Can you work these out from the model? Positions are in its coordinate system, mm. Face numbers are marked on the shaded views. A direction names the side the tool comes from. Give positions to 0.01 mm unless a question says otherwise; leave off trailing zeros. Loops run counter-clockwise (first coordinate to the right, second up) from the corner with the lowest first, then second, coordinate; pieces in that order, holes last. Notation, with made-up numbers: M 54.5,74.5 L 71.5,74.5 A35 ccw 71.5,110.5 Z; hole C 70.25,19 d8. An arc over 180 degrees is marked long. Put each result on its own line as item: value. Start each with the question number.
1) For the marked faces 5, 6 and 7, which set-ups out of +Z, -Z, +X, -X, +Y, -Y let a thin tool reach every point of the face, with its end or its side?
2) Please list where these lines run through material, in increasing order: line 1 along Y through (x, z) = (15, 7); line 2 along X through (y, z) = (58.75, 2.75); line 3 along X through (y, z) = (58.25, 8.5). Write a range as from..to.
3) Imagine slicing it at C-C (z = 15). State how many separate pieces and enclosed holes the cut face has, then the cut area to 3 significant figures.
4) Imagine slicing it at B-B (x = 15). Write out the boundary of the cut face in (y, z), then the cut area to 3 significant figures.
5) Imagine slicing it at A-A (x = -15). Write out the boundary of the cut face in (y, z), then the cut area to 3 significant figures.
6) Imagine slicing it at D-D (x = -9). Write out the boundary of the cut face in (y, z).
7) If we mould it in two halves opening along Y, with no side actions, what happens to the marked faces 1, 2, 3 and 4? For each: +Y half, -Y half, draft (parallel to the pull), parting line (faces both ways), or undercut.
8) For P1, Ø5, axis at x = 17.5, z = 11, coming from the +Y side; P2, Ø8, axis at x = 13, y = 59.5, coming from the -Z side; P3, Ø8, axis at x = 26, y = 58, coming from the +Z side; P4, Ø4, axis at x = 12.5, z = 6, coming from the -Y side, each with a flat end and sliding along its axis, tell me the tip position at first contact or that it passes through.
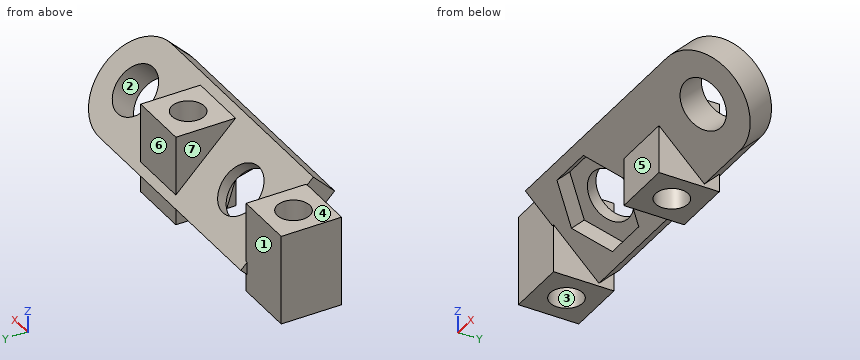
from build123d import *

# Parameters (mm, degrees)
SKETCH039_R             = 4.2
PAD019_DEPTH            = 5
BOX_W                   = 10
BOX_H                   = 10
BOX_DEPTH               = 15
POCKET011_DEPTH         = 3
SKETCH041_R             = 2.7
POCKET012_DEPTH         = 130.641501891
BODY007_PLACEMENT_ANGLE = 45


with BuildPart() as part:
    # Sketch039 → Pad019 (new body)
    with BuildSketch(Plane.XZ):
        with BuildLine():
            ThreePointArc((30, -8.5), (38.5, 0), (30, 8.5))
            Line((0, 8.5), (30, 8.5))
            Line((-10.313604, 8.5), (0, 8.5))
            Line((-10.313604, -8.5), (-10.313604, 8.5))
            Line((0, -8.5), (-10.313604, -8.5))
            Line((0, -8.5), (30, -8.5))
        make_face()
        Circle(SKETCH039_R, mode=Mode.SUBTRACT)
        with Locations((30, 0)):
            Circle(SKETCH039_R, mode=Mode.SUBTRACT)
    extrude(amount=PAD019_DEPTH)

    # Box → Box (join)
    with BuildSketch(Plane(origin=(10, 7, 0), x_dir=(1, 0, 0), z_dir=(0, -0.7071067812, -0.7071067812))):
        with Locations((5, 5)):
            Rectangle(BOX_W, BOX_H)
    box = extrude(amount=BOX_DEPTH)

    # Sketch040 (on Face5 of Box) → Pocket011 (cut)
    with BuildSketch(Plane(origin=(10, -5, 0), x_dir=(1, 0, 0), z_dir=(0, -1, 0))):
        Polygon((-6.2472232503, 6.5), (-13.7527767497, 6.5), (-17.5055534995, 0), (-13.7527767497, -6.5), (-6.2472232503, -6.5), (-2.4944465005, 0), align=None)
    extrude(amount=-POCKET011_DEPTH, mode=Mode.SUBTRACT)

    # Sketch041 (on Face15 of Pocket011) → Pocket012 (cut, through all)
    with BuildSketch(Plane(origin=(10, 7, 0), x_dir=(1, 0, 0), z_dir=(0, 0.7071067812, 0.7071067812))):
        with Locations((5, -4.9497474683)):
            Circle(SKETCH041_R)
    pocket012 = extrude(amount=-POCKET012_DEPTH, mode=Mode.SUBTRACT)

    # Mirrored010: Box, Pocket012 across YZ
    add(box.mirror(Plane.YZ))
    add(pocket012.mirror(Plane.YZ), mode=Mode.SUBTRACT)


with BuildPart() as part_1:
    # Body007 placement: moved
    add(part.part.moved(Location((0, 59, 11))).rotate(Axis((0, 59, 11), (1, 0, 0)), BODY007_PLACEMENT_ANGLE))


solid = part_1.part
Recorded:
1. face 5: -Z, +X, -X, -Y
1. face 6: +Z, +X, -X, +Y
1. face 7: +Z, +Y
2. line 1: 53.95..56.3, 61.7..63.95
2. line 2: -20..-17.69, -12.31..-10, 10..12.31, 17.69..20
2. line 3: -20..-17.59, -12.41..-6.79, 6.79..12.41, 17.59..25.99, 34.01..38.41
3. separate pieces: 1
3. enclosed holes: 2
3. area: 323 mm²
4. outline: M 49.45,13.47 L 53.95,8.98 L 53.95,0.95 L 56.3,0.95 L 56.3,15.95 L 54.05,15.95 L 52.99,17.01 Z; M 61.7,0.95 L 63.95,0.95 L 63.95,3.93 L 65.01,4.99 L 63.95,6.05 L 63.95,15.95 L 61.7,15.95 Z
4. area: 89.4 mm²
5. outline: M 53.95,0.95 L 56.3,0.95 L 56.3,15.95 L 53.95,15.95 Z; M 61.7,0.95 L 63.95,0.95 L 63.95,15.95 L 61.7,15.95 Z
5. area: 69.0 mm²
6. outline: M 49.45,13.47 L 61.47,1.45 L 65.01,4.99 L 52.99,17.01 Z
7. face 1: +Y half
7. face 2: undercut
7. face 3: undercut
7. face 4: draft
8. P1: y = 63.95
8. P2: z = 0.95
8. P3: z = 16
8. P4: y = 53.95
